Part model, mm, in its own coordinate system. A direction names the side the tool comes from. Round coordinates to 2 decimals unless told otherwise and drop trailing zeros.
(1) Probe probe 1 along Z at (x, y) = (7, 113); probe 2 along X at (y, z) = (-98, -66.5); probe 3 along X at (y, z) = (6.5, -38.5). List the from-to ranges inside material, lowest first.
(2) Flat gauge pins, fed straight in: pin 1 (2 mm diameter, centred on y = -66.5, z = 46.5, fed in from -X); pin 2 (2 mm diameter, centred on y = -15.5, z = 19.5, fed in from +X); pin 3 (3 mm diameter, centred on x = -58.5, z = 93.5, fed in from +Y). Where does each tip first touch, or does it go through?
(3) Mould opens along Y. For faces 1 (the face through (9.396, 30.093, 118.525)), 2 (the face through (-215.673, -99.304, -96.071)) say: +Y half, -Y half, draft (parallel to the pull), parting line (faces both ways), or undercut.
(4) Tool access for faces 3 (the face through (-122.8, -165.1, -80.7)), 4 (the face through (-121.074, -157.213, 32.03)): list every direction of +Z, -Z, +X, -X, +Y, -Y with a clear straight run to the whole face (end or side of a thin tool).
from build123d import *


with BuildPart() as f1:
    # F0 (on Front) → F1 (revolve)
    with BuildSketch(Plane.XZ):
        Polygon((-83.341058, 21.032826), (-86.163277, 17.317339), (-86.163277, -16.894962), (-83.511949, -20.046823), (-80.697984, -23.491596), (-77.732458, -27.199996), (-74.620857, -31.141314), (-71.371333, -35.289109), (-67.993895, -39.6145), (-64.493775, -44.089218), (-60.881641, -48.682021), (-57.162319, -53.367559), (-53.345207, -58.116343), (-49.438687, -62.899417), (-45.449109, -67.686834), (-41.386887, -72.451849), (-37.256847, -77.166343), (-33.069149, -81.799049), (-28.830143, -86.324846), (-24.548465, -90.712442), (-20.232497, -94.933389), (-15.888843, -98.961321), (-11.525885, -102.764742), (-7.152259, -106.317161), (-2.774315, -109.588681), (1.598549, -112.551591), (5.958459, -115.176706), (10.299319, -117.4353), (14.611477, -119.299761), (18.887313, -120.741211), (23.119207, -121.730668), (27.300047, -122.239126), (31.420435, -122.237779), (35.474529, -121.698918), (39.453185, -120.595111), (42.453179, -119.090313), (45.210603, -117.837661), (47.753143, -116.789022), (50.114835, -115.891894), (52.322603, -115.096773), (54.408959, -114.35273), (56.403113, -113.609755), (58.337831, -112.817554), (60.240799, -111.927284), (62.144021, -110.885351), (64.077215, -109.645323), (66.071369, -108.154114), (68.156455, -106.361382), (70.363969, -104.218359), (72.723121, -101.674549), (75.266931, -98.678873), (76.934441, -96.262825), (78.564613, -93.191203), (80.121887, -89.559003), (81.571465, -85.461983), (82.881851, -80.995926), (84.020279, -76.258039), (84.950427, -71.344155), (85.639529, -66.350286), (86.055581, -61.372648), (86.163277, -56.508015), (85.930359, -51.851687), (85.322537, -47.49993), (84.306791, -43.550484), (82.848831, -40.097075), (80.915637, -37.236298), (78.473681, -35.067367), (76.249403, -33.573339), (73.435591, -31.652337), (70.133591, -29.375989), (66.443479, -26.81544), (62.466347, -24.043005), (58.303287, -21.132673), (54.057677, -18.155818), (49.828577, -15.184755), (45.717841, -12.292203), (41.826053, -9.551568), (38.255575, -7.032371), (35.108007, -4.809617), (32.483171, -2.95468), (30.483429, -1.54117), (29.208857, -0.638175), (28.762325, -0.322453), (29.302329, 0.020447), (30.833441, 0.997585), (33.223327, 2.532482), (36.334827, 4.550004), (40.034591, 6.973951), (44.188253, 9.728835), (48.662463, 12.736957), (53.321585, 15.922879), (58.030491, 19.211138), (62.657863, 22.525076), (67.067557, 25.789763), (71.124699, 28.927654), (74.695177, 31.864148), (77.645387, 34.522283), (79.840709, 36.825022), (81.147031, 38.697789), (83.936205, 45.91873), (85.235669, 53.169947), (85.211031, 60.370339), (84.027137, 67.435603), (81.847309, 74.28291), (78.838679, 80.828769), (75.165077, 86.991038), (70.990841, 92.686505), (68.214113, 96.146976), (65.900427, 99.029622), (63.975107, 101.408357), (62.360175, 103.356791), (60.979431, 104.94833), (59.756929, 106.256201), (58.617485, 107.355742), (57.483375, 108.317919), (56.277637, 109.218832), (54.924325, 110.129701), (53.349271, 111.126397), (51.473735, 112.279557), (49.223549, 113.665889), (46.519719, 115.355751), (43.288331, 117.425851), (39.453185, 119.948071), (36.213415, 121.253606), (32.813625, 122.007986), (29.266769, 122.239126), (25.583007, 121.974991), (21.774277, 121.235826), (17.850993, 120.052186), (13.827125, 118.446906), (9.712325, 116.450466), (5.517515, 114.081941), (1.256665, 111.371507), (-3.060573, 108.345351), (-7.420737, 105.026816), (-11.815191, 101.443917), (-16.230473, 97.619922), (-20.655407, 93.583633), (-25.077547, 89.359867), (-29.487241, 84.973795), (-33.872297, 80.452341), (-38.220015, 75.819102), (-42.519473, 71.102347), (-46.759749, 66.327376), (-50.928397, 61.517886), (-55.015257, 56.703316), (-59.006359, 51.907542), (-62.892559, 47.155989), (-66.661411, 42.474998), (-70.301993, 37.890323), (-73.800919, 33.428051), (-77.148182, 29.113607), (-80.332809, 24.974169), align=None)
    revolve(axis=Axis((-86.163277, 0, 0.211188), (0, 0, 1)))


solid = f1.part
Final values:
1. probe 1: z = -111.9 to -22.52, 20.83 to 105.69
1. probe 2: x = -227.25 to 54.92
1. probe 3: x = -253.97 to -102.19, -70.13 to 81.64
2. pin 1: stops at x = -243.3
2. pin 2: stops at x = 59.01
2. pin 3: stops at y = 155.24
3. face 1: undercut
3. face 2: parting line
4. face 3: -Z
4. face 4: none
